Build history of the part. All positions in model axes, mm. A direction names the side the tool comes from. Give positions to 0.01 mm unless a question says otherwise; leave off trailing zeros. Loops run counter-clockwise (first coordinate to the right, second up) from the corner with the lowest first, then second, coordinate; pieces in that order, holes last. Notation, with made-up numbers: M -12,1.5 L 17,1.5 A10 cw 17,20.5 Z; hole C 0,70.5 d8. An arc over 180 degrees is marked long. Put each result on its own line as item: value.
Autodesk Inventor part; units mm, degrees
ref_plane "YZ Plane" through (0, 0, 0) normal (1, 0, 0) x (0, 1, 0)
ref_plane "XZ Plane" through (0, 0, 0) normal (0, 1, 0) x (-1, 0, 0)
ref_plane "XY Plane" through (0, 0, 0) normal (0, 0, 1) x (1, 0, 0)
sketch "Sketch1" plane through (0, 0, 0) normal (0, 0, 1) x (1, 0, 0)
  line L0 (3.175, 0) -> (3.175, 3.175)
  line L1 (3.175, 3.175) -> (-3.175, 3.175)
  line L2 (-3.175, 3.175) -> (-3.175, 0)
  line L3 (5.08, 0) -> (5.08, 5.08)
  line L4 (5.08, 5.08) -> (-5.08, 5.08)
  line L5 (-5.08, 5.08) -> (-5.08, 0)
  line L6 (-5.08, 0) -> (-3.175, 0)
  line L7 (3.175, 0) -> (5.08, 0)
  point P0 (0, 0)
  dimension "d0" = 10.16
  dimension "d1" = 5.08
extrude "Extrusion1" add sketch "Sketch1" along normal blind 215.9
sketch "Sketch2" plane through (-5.08, 5.08, 0) normal (0, 1, 0) x (1, 0, 0)
  circle A0 centre (5.08, -6.35) radius 1.9844
  circle A1 centre (5.08, -209.55) radius 1.9844
  point P0 (5.08, 0)
  dimension "d4" = 3.9688
  dimension "d5" = 3.9688
extrude "Extrusion2" cut sketch "Sketch2" against normal blind 215.9
sketch "Sketch3" plane through (-5.08, 5.08, 0) normal (0, 1, 0) x (1, 0, 0)
  circle A0 centre (5.08, -6.35) radius 1.9844
  circle A1 centre (5.08, -209.55) radius 1.9844
  circle A2 centre (5.08, -209.55) radius 5.08
  line L0 (10.16, 0) -> (10.16, -215.9)
  circle A3 centre (5.08, -6.35) radius 5.08
  point P0 (5.08, 0)
extrude "Extrusion3" add sketch "Sketch3" along normal blind 12.7
sketch "Sketch4" plane through (0, 0, 215.9) normal (0, 0, 1) x (1, 0, 0)
  line L0 (-5.08, 5.08) -> (-5.08, 0)
  line L1 (-5.08, 0) -> (5.08, 0)
  line L2 (5.08, 0) -> (5.08, 5.08)
  line L3 (5.08, 5.08) -> (-5.08, 5.08)
  line L4 (-5.08, 5.08) -> (-5.08, 0)
  point P0 (0, 0)
extrude "Extrusion4" add sketch "Sketch4" along normal blind 5.08
properties part number "bumper"
Q1. Drop flat-ended pins along their axis: pin 1 Ø4.5 at (x, z) = (0, 209.55) entering from +Y; pin 2 Ø3 at (x, z) = (0.5, 217) entering from +Y; pin 3 Ø3.5 at (x, y) = (-1, 1) entering from -Z; pin 4 Ø1.5 at (x, y) = (1, 14) entering from -Z. Give the stop position or say it passes through.
Here are the results:
pin 1: y = 17.78
pin 2: y = 5.08
pin 3: z = 215.9
pin 4: z = 1.28
Q2. Probe line 1 (Z direction, x = -0.25, y = 4.25); line 2 (Z direction, x = 0, y = 10.5); line 3 (X direction, y = 13, z = 6.35). List the from-to ranges inside material, lowest first. Write a range as from..to.
Here are the results:
line 1: 0..4.38, 8.32..207.58, 211.52..220.98
line 2: 1.27..4.37, 8.33..11.43, 204.47..207.57, 211.53..214.63
line 3: -5.08..-1.98, 1.98..5.08
Q3. Mould opens along X. For faces 1 (the flat face through (0, 3.175, 106)), 2 (the cylindrical face through (-0.661, 11.341, 214.587)), 3 (the flat face through (-5.08, 3, 109)), 4 (the flat face through (0, 4, 0)) say: pulls with the +X half, pulls with the -X half, needs draft (parallel to the pull), parting line crosses it, or undercut.
Here are the results:
face 1: undercut
face 2: parting line crosses it
face 3: pulls with the -X half
face 4: needs draft
Q4. Slice it at B-B (y = 9.5). List the corners of the cut face in (x, z).
Here are the results:
outline: C 0,6.35 d10.16; C 0,209.55 d10.16; hole C 0,6.35 d3.97; hole C 0,209.55 d3.97
Q5. Tool access for faces 5 (the cylindrical face through (-0.258, 10.58, 4.382)), 6 (the flat face through (0, 5.08, 1)), 7 (the cylindrical face through (-1.1, 11.34, 1.39)): list every direction of +Z, -Z, +X, -X, +Y, -Y with a clear straight run to the whole face (end or side of a thin tool).
Here are the results:
face 5: +Y, -Y
face 6: -Z, +Y
face 7: +Y
Q6. Slice it at A-A (x = 0). List the corners of the cut face in (y, z) (3 decimals).
Here are the results:
outline: M 0,215.9 L 3.175,215.9 L 3.175,211.534 L 17.78,211.534 L 17.78,214.63 L 5.08,214.63 L 5.08,220.98 L 0,220.98 Z; M 3.175,0 L 5.08,0 L 5.08,1.27 L 17.78,1.27 L 17.78,4.366 L 3.175,4.366 Z; M 3.175,8.334 L 17.78,8.334 L 17.78,11.43 L 5.08,11.43 L 5.08,204.47 L 17.78,204.47 L 17.78,207.566 L 3.175,207.566 Z
Q7. Slice it at C-C (z = 85.5). List the corners of the cut face in (x, y) (3 decimals).
Here are the results:
outline: M -5.08,0 L -3.175,0 L -3.175,3.175 L 3.175,3.175 L 3.175,0 L 5.08,0 L 5.08,5.08 L -5.08,5.08 Z
